Work out the finished part from the listing and answer in its coordinate system (mm). A direction names the side the tool comes from. Round coordinates to 2 decimals unless told otherwise and drop trailing zeros. Write each loop counter-clockwise with the first axis right and the second up, starting at its lowest first coordinate (ties: lowest second). Pieces come first, ordered by that corner, then holes. Notation, with made-up numbers: (72, -3.75) - (127, -3.75) arc R24 cw to (127, 19.25) - close; hole circle Ø4 at (75.25, -36). An arc over 180 degrees is marked (long way). Answer as a JSON object with one key per item and string values.
```python
from build123d import *

# Parameters (mm, degrees)
F3_ANGLE = 90


with BuildPart() as f1:
    # F0 (on Top) → F1 (revolve)
    with BuildSketch(Plane.XY):
        with BuildLine():
            Line((0, 8.9), (0, 7.9))
            Line((0, 7.9), (2.4, 7.9))
            Line((2.4, 7.9), (2.4, 6.8))
            Line((2.4, 6.8), (5.4, 6.8))
            Line((5.4, 6.8), (5.4, 7.9))
            ThreePointArc((5.4, 7.9), (9.5153331571, 6.7434437053), (12.4257006262, 3.6124134192))
            Line((12.4257006262, 3.6124134192), (13.0271804842, 2.4426089354))
            Line((13.0271804842, 2.4426089354), (17.9327297956, 0.6101466133))
            Line((17.9327297956, 0.6101466133), (20.8739452064, 0))
            Line((20.8739452064, 0), (25.4, 0))
            ThreePointArc((25.4, 0), (19.537082279, 0.996970145), (13.951692761, 3.0393162482))
            ThreePointArc((13.951692761, 3.0393162482), (10.617032549, 7.3430021373), (5.4, 8.9))
            Line((5.4, 8.9), (0, 8.9))
        make_face()
    revolve(axis=Axis((12.5827532146, 0, 0), (1, 0, 0)))


with BuildPart() as f1_1:
    # F3: moved
    add(f1.part.rotate(Axis((0, 0, 0), (0, -1, 0)), F3_ANGLE))


solid = f1_1.part
```
Item 1: Determine the mould class of faces 1 (the cylindrical face through (8.69, -1.93, 2.66)), 2 (the flat face through (8, -1, 0)), 3 (the flat face through (-6, -4, 2.4)), 4 (the cylindrical face through (6.64, -1.47, 3.92)) for opening direction Y: pulls with the +Y half, pulls with the -Y half, needs draft (parallel to the pull), parting line crosses it, or undercut.
Results found:
{"face 1": "parting line crosses it", "face 2": "needs draft", "face 3": "undercut", "face 4": "undercut"}
Item 2: Consider line 1 along X through (y, z) = (0, 1.45); line 2 along X through (y, z) = (0, 3.05); line 3 along Y through (x, z) = (-2.75, 11). Determine where each line is inside the solid, lowest interval first.
Results found:
{"line 1": "-8.9 to -7.9, 7.9 to 8.9", "line 2": "-8.9 to -6.8, 6.8 to 8.9", "line 3": "-6.51 to -4.85, 4.85 to 6.51"}
Item 3: A cutting plane is placed at A-A (z = 3). Write down the section's boundary in (x, y), and give its area (3 significant figures).
Results found:
{"outline": "circle Ø17.8 at (0, 0); hole circle Ø13.6 at (0, 0)", "area": "104 mm²"}
Item 4: For faces 5 (the flat face through (-6, 4, 5.4)), 6 (the cylindrical face through (4.807, -6.269, 1.217)), determine the directions among +Z, -Z, +X, -X, +Y, -Y from which every point of the face is accessible in a straight line to the end or side of a thin tool.
Results found:
{"face 5": "none", "face 6": "-Z"}
Item 5: A cutting plane is placed at C-C (z = 7). Write down the section's boundary in (x, y), and give its area (3 significant figures).
Results found:
{"outline": "circle Ø17.58 at (0, 0); hole circle Ø15.47 at (0, 0)", "area": "54.6 mm²"}
Item 6: Each of these flat-tipped pins is pushed along its axis until it touches: P1, Ø4.5, axis at x = -2, y = 0.5, coming from the -Z side; P2, Ø8, axis at x = 1.5, z = 21.5, coming from the -Y side; P3, Ø1.5, axis at y = 0, z = 8, coming from the -X side. Where does it stop, or does it pass through?
Results found:
{"P1": "z = 12.02", "P2": "y = -1.52", "P3": "x = -8.74"}
